Check sheet for the modelled part. Datum: model origin and axes. Units: mm. A direction names the side the tool comes from. Round coordinates to 2 decimals unless told otherwise and drop trailing zeros. Loops run counter-clockwise (first coordinate to the right, second up) from the corner with the lowest first, then second, coordinate; pieces in that order, holes last. Notation, with made-up numbers: (-6.5, 54) - (48.5, 54) arc R20 ccw to (48.5, 59) - close; hole circle Ø6 at (-5, 17.5). An arc over 180 degrees is marked (long way). Put each result on its own line as item: value. Start each with the question number.
```python
from build123d import *

# Parameters (mm, degrees)
SKETCH1_R               = 4.445
BOSS_EXTRUDE1_DEPTH     = 28.575
SKETCH2_R               = 6.35
SKETCH2_R_2             = 3.81
CUT_EXTRUDE_THIN1_DEPTH = 14.605


with BuildPart() as part:
    # Sketch1 → Boss-Extrude1 (new body, symmetric)
    with BuildSketch(Plane(origin=(0, 0, 0), x_dir=(0, 0, -1), z_dir=(1, 0, 0))):
        Circle(SKETCH1_R)
    extrude(amount=BOSS_EXTRUDE1_DEPTH, both=True)

    # Sketch2 → Cut-Extrude-Thin1 (cut)
    with BuildSketch(Plane(origin=(28.575, 0, 0), x_dir=(0, 0, -1), z_dir=(1, 0, 0))):
        Circle(SKETCH2_R)
        Circle(SKETCH2_R_2, mode=Mode.SUBTRACT)
    cut_extrude_thin1 = extrude(amount=-CUT_EXTRUDE_THIN1_DEPTH, mode=Mode.SUBTRACT)

    # Mirror1: Cut-Extrude-Thin1 across plane
    add(cut_extrude_thin1.mirror(Plane(origin=(0, 0, 0), x_dir=(0, 0, 1), z_dir=(1, 0, 0))), mode=Mode.SUBTRACT)


solid = part.part
```
Q1. Depth check by flat-ended pin: pin 1 Ø5 at (x, z) = (-4, -1) entering from +Y (3 decimals); pin 2 Ø2 at (x, z) = (-20.5, 3) entering from -Y; pin 3 Ø4 at (x, z) = (-9.5, -3) entering from +Y. Enter the tip coordinate at first touch or a pass-through.
Q2. Material ranges on line 1 (Y direction, x = 19, z = 0.25); line 2 (X direction, y = -3.25, z = 2.25); line 3 (Z direction, x = 21.5, y = 1.5), recorded low to high. Write a range as from..to.
Q3. Set-up check for faces 1 (the face through (-13.97, 1, -4)), 2 (the face through (-28.575, 0, 0)), 3 (the face through (13.97, 1, -4)): record each of +Z, -Z, +X, -X, +Y, -Y from which the full face is reachable in a straight line by a thin tool's end or side.
Q4. Cross-section at A-A on z = 0. Enter the section's corners in (x, y) (3 decimals), and give its area (3 significant figures).
Q5. Cross-section at D-D on x = 0. Enter the section's corners in (y, z) (3 decimals), and give its area (3 significant figures).
Q6. Cross-section at C-C on x = -21.5. Enter the section's corners in (y, z).
Answer list:
1. pin 1: stops at y = 4.445
1. pin 2: stops at y = -3.24
1. pin 3: stops at y = 4.33
2. line 1: y = -3.8..3.8
2. line 2: x = -13.97..13.97
2. line 3: z = -3.5..3.5
3. face 1: -X
3. face 2: +Z, -Z, -X, +Y, -Y
3. face 3: +X
4. outline: (-28.575, -3.81) - (-13.97, -3.81) - (-13.97, -4.445) - (13.97, -4.445) - (13.97, -3.81) - (28.575, -3.81) - (28.575, 3.81) - (13.97, 3.81) - (13.97, 4.445) - (-13.97, 4.445) - (-13.97, 3.81) - (-28.575, 3.81) - close
4. area: 471 mm2
5. outline: circle Ø8.89 at (0, 0)
5. area: 62.1 mm2
6. outline: circle Ø7.62 at (0, 0)
